from build123d import *

# Parameters (mm, degrees)
SKETCH1_W           = 53.5
SKETCH1_H           = 60
SKETCH1_W_2         = 45.5
SKETCH1_H_2         = 52
BOSS_EXTRUDE1_DEPTH = 47
CUT_EXTRUDE1_START  = -4
SKETCH3_R           = 1.5
CUT_EXTRUDE1_DEPTH  = 82.273863628
LPATTERN1_COUNT     = 2
LPATTERN1_PITCH     = 28.7
SKETCH4_R           = 1.5
CUT_EXTRUDE2_DEPTH  = 4
LPATTERN2_COUNT     = 2
LPATTERN2_PITCH     = 28.7
SKETCH5_W           = 15
SKETCH5_H           = 15
SKETCH5_W_2         = 12.5
SKETCH5_H_2         = 12.5
BOSS_EXTRUDE2_DEPTH = 17
SKETCH6_R           = 1.5
CUT_EXTRUDE3_DEPTH  = 60.742904181


with BuildPart() as part:
    # Sketch1 → Boss-Extrude1 (new body)
    with BuildSketch(Plane(origin=(0, 0, 0), x_dir=(1, 0, 0), z_dir=(0, 1, 0))):
        Rectangle(SKETCH1_W, SKETCH1_H)
        Rectangle(SKETCH1_W_2, SKETCH1_H_2, mode=Mode.SUBTRACT)
    extrude(amount=BOSS_EXTRUDE1_DEPTH)

    # Sketch3 → Cut-Extrude1 (cut)
    with BuildSketch(Plane.ZY.offset(26.75).offset(CUT_EXTRUDE1_START)):
        with Locations(Location((18, 30.05, 0), (0, 0, 180))):
            Circle(SKETCH3_R)
        with Locations(Location((11, 20.05, 0), (0, 0, 180))):
            Circle(SKETCH3_R)
    cut_extrude1 = extrude(amount=CUT_EXTRUDE1_DEPTH, mode=Mode.SUBTRACT)

    # LPattern1: Cut-Extrude1 ×2
    with Locations(*[(0, 0, -i * LPATTERN1_PITCH) for i in range(1, LPATTERN1_COUNT)]):
        add(cut_extrude1, mode=Mode.SUBTRACT)

    # Sketch4 → Cut-Extrude2 (cut)
    with BuildSketch(Plane(origin=(26.75, 0, 0), x_dir=(0, 0, -1), z_dir=(1, 0, 0))):
        with Locations((-11, 30.05)):
            Circle(SKETCH4_R)
        with Locations((-18, 20.05)):
            Circle(SKETCH4_R)
    cut_extrude2 = extrude(amount=-CUT_EXTRUDE2_DEPTH, mode=Mode.SUBTRACT)

    # LPattern2: Cut-Extrude2 ×2
    with Locations(*[(0, 0, -i * LPATTERN2_PITCH) for i in range(1, LPATTERN2_COUNT)]):
        add(cut_extrude2, mode=Mode.SUBTRACT)

    # Sketch5 → Boss-Extrude2 (add)
    # profile 1 of 2: a face of its own
    with BuildSketch(Plane.XY.offset(30)):
        with Locations((-15, 14.11)):
            Rectangle(SKETCH5_W, SKETCH5_H)
        with Locations((-15, 14.11)):
            Rectangle(SKETCH5_W_2, SKETCH5_H_2, mode=Mode.SUBTRACT)
    # profile 2 of 2: a face of its own
    with BuildSketch(Plane.XY.offset(30)):
        with Locations((15, 14.11)):
            Rectangle(SKETCH5_W, SKETCH5_H)
        with Locations((15, 14.11)):
            Rectangle(SKETCH5_W_2, SKETCH5_H_2, mode=Mode.SUBTRACT)
    extrude(amount=BOSS_EXTRUDE2_DEPTH)

    # Sketch6 → Cut-Extrude3 (cut, through all)
    with BuildSketch(Plane(origin=(0, 21.61, 0), x_dir=(1, 0, 0), z_dir=(0, 1, 0))):
        with Locations(Location((-15, -38.5, 0), (0, 0, 270))):
            Circle(SKETCH6_R)
        with Locations(Location((15, -38.5, 0), (0, 0, 270))):
            Circle(SKETCH6_R)
    extrude(amount=-CUT_EXTRUDE3_DEPTH, mode=Mode.SUBTRACT)


solid = part.part
Verification items for the finished model (mm, model axes). A direction names the side the tool comes from. Round coordinates to 2 decimals unless told otherwise and drop trailing zeros. Order: outer loops, then holes, each group sorted by start corner. A loop starts at its lowest first (then second) coordinate and runs counter-clockwise, first axis right, second up.
1. Section check C-C on x = -1. Record the cut outline in (y, z).
Final values:
outline: (0, -30) - (47, -30) - (47, -26) - (0, -26) - close; (0, 26) - (47, 26) - (47, 30) - (0, 30) - close
2. Thickness scan on L1, parallel to X at y = 7.1, z = 38.5; L2, parallel to Z at x = 24, y = 20; L3, parallel to Z at x = 23, y = 30. Record the ranges inside material, lowest first.
Final values:
L1: x = -22.5 to -16.5, -13.5 to -7.5, 7.5 to 13.5, 16.5 to 22.5
L2: z = -30 to -12.2, -9.2 to 16.5, 19.5 to 30
L3: z = -30 to -19.2, -16.2 to 9.5, 12.5 to 30
3. Section check A-A on z = 38.5. State how many separate pieces and enclosed holes the cut face has, then the cut area to 4 significant figures.
Final values:
separate pieces: 4
enclosed holes: 0
area: 122.5 mm2
4. Release check for a two-part mould opening along Z. For faces 1 (the cylindrical face through (-15.9, 21, 37.3)), 2 (the flat face through (-24, 47, 0)), 3 (the flat face through (8, 14, 47)) record: +Z half, -Z half, draft (parallel to the pull), parting line (faces both ways), or undercut.
Final values:
face 1: undercut
face 2: draft
face 3: +Z half
5. Section check B-B on y = 30.05. Record the cut outline in (x, z), then the cut area to 3 significant figures.
Final values:
outline: (-26.75, -30) - (26.75, -30) - (26.75, -19.2) - (22.75, -19.2) - (22.75, -26) - (-22.75, -26) - (-22.75, -12.2) - (-26.75, -12.2) - close; (-26.75, -9.2) - (-22.75, -9.2) - (-22.75, 16.5) - (-26.75, 16.5) - close; (-26.75, 19.5) - (-22.75, 19.5) - (-22.75, 26) - (22.75, 26) - (22.75, 12.5) - (26.75, 12.5) - (26.75, 30) - (-26.75, 30) - close; (22.75, -16.2) - (26.75, -16.2) - (26.75, 9.5) - (22.75, 9.5) - close
area: 796 mm2
6. Access from +Z, -Z, +X, -X, +Y, -Y to the whole of each face (thin tool, end or side, straight path). Record for faces 4 (the flat face through (8.75, 14, 38)), 5 (the cylindrical face through (24.778, 18.586, -10.375)), 6 (the flat face through (-13, 6.61, 38)).
Final values:
face 4: +Z
face 5: +X
face 6: +Z, +X, -X, -Y
7. Section check D-D on y = 25. Record the cut outline in (x, z).
Final values:
outline: (-26.75, -30) - (26.75, -30) - (26.75, 30) - (-26.75, 30) - close; hole (-22.75, -26) - (22.75, -26) - (22.75, 26) - (-22.75, 26) - close
8. Go/stop test with flat-tipped pins: P1, Ø12, axis at y = 13.5, z = 35.5, coming from the +X side; P2, Ø4, axis at y = 16.5, z = 41.5, coming from the +X side; P3, Ø10, axis at x = 16, z = 41, coming from the +Y side; P4, Ø5, axis at x = 10.5, y = 33, coming from the +Z side. Record where each tip stops, or that it passes through.
Final values:
P1: stops at x = 26.75
P2: stops at x = 22.5
P3: stops at y = 21.61
P4: stops at z = 30
